The listing builds one solid part. Answer for the finished solid, in the listing's coordinates (mm). Face numbers are marked on the shaded views. A direction names the side the tool comes from. Round coordinates to 2 decimals unless told otherwise and drop trailing zeros. Write each loop counter-clockwise with the first axis right and the second up, starting at its lowest first coordinate (ties: lowest second). Pieces come first, ordered by that corner, then holes.
Item 1: Each of these flat-tipped pins is pushed along its axis until it touches: pin 1 (2 mm diameter, centred on x = 4, y = 13, fed in from -Z); pin 2 (1 mm diameter, centred on x = 2, y = 10, fed in from +Z); pin 3 (1.5 mm diameter, centred on x = -3, y = 2.5, fed in from +Z). Where does it stop, or does it pass through?
Item 2: Find section B-B on z = -5.5. Give the vertices of the cut face in (x, y), then the cut area to 3 significant figures.
Item 3: For a pull along Z with two mould halves and no side action, classify the marked faces 4 and 5 as +Z half, -Z half, draft (parallel to the pull), parting line (faces both ways), or undercut.
Item 4: Find section D-D on z = 0. Give the vertices of the cut face in (x, y).
Item 5: Find section C-C on x = 0. Give the vertices of the cut face in (y, z).
Item 6: Find section A-A on x = -4.25. Give the vertices of the cut face in (y, z), then the cut area to 3 significant figures.
Item 7: Find the intervals of material crossed by probe 1 along X at (y, z) = (10.5, -6.25); probe 2 along X at (y, z) = (7.75, -7); probe 3 along Z at (x, y) = (-6.5, 3), in increasing order.
Item 8: A tool of negligible diameter and unlimited length cuts with its end or side. For the marked faces 1, 2 and 3, from which of +Z, -Z, +X, -X, +Y, -Y can it reach the whole face along a straight path? Write none if from no direction.
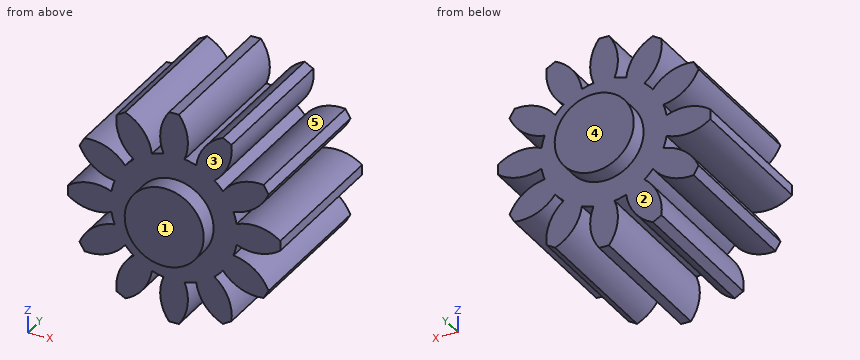
```python
from build123d import *

# Parameters (mm, degrees)
BOSS_EXTRUDE2_DEPTH = 12.5
CIRPATTERN1_COUNT   = 12


with BuildPart() as part:
    # Sketch1 → Revolve1 (revolve)
    with BuildSketch(Plane(origin=(0, 0, 0), x_dir=(0, 0, -1), z_dir=(1, 0, 0)), mode=Mode.PRIVATE) as revolve1_sk:
        Polygon((0, 0), (3.2, 0), (3.2, 1.5), (5.13, 1.5), (5.13, 14), (3.2, 14), (3.2, 15.5), (0, 15.5), align=None)
    revolve(revolve1_sk.sketch.rotate(Axis((0, 15.5, 0), (0, -1, 0)), 180), axis=Axis((0, 15.5, 0), (0, -1, 0)))

    # Sketch2 → Boss-Extrude2 (add)
    with BuildSketch(Plane(origin=(0, 14, 0), x_dir=(1, 0, 0), z_dir=(0, 1, 0))):
        with BuildLine():
            Line((0.4, 8.6), (-0.4, 8.6))
            ThreePointArc((-0.4, 8.6), (-1.094743674, 6.889243261), (-0.85, 5.059090827))
            Line((-0.85, 5.059090827), (-0.85, 4.768997596))
            Line((-0.85, 4.768997596), (0.85, 4.768997596))
            Line((0.85, 4.768997596), (0.85, 5.059090827))
            ThreePointArc((0.85, 5.059090827), (1.094743674, 6.889243261), (0.4, 8.6))
        make_face()
    boss_extrude2 = extrude(amount=-BOSS_EXTRUDE2_DEPTH)

    # CirPattern1: Boss-Extrude2 ×12 about axis
    cirpattern1_axis = Axis((0, 0, 0), (0, 1, 0))
    for i in range(1, CIRPATTERN1_COUNT):
        add(boss_extrude2.rotate(cirpattern1_axis, i * 360 / CIRPATTERN1_COUNT))


solid = part.part
```
Check values:
1. pin 1: stops at z = -7.65
1. pin 2: stops at z = 6.52
1. pin 3: stops at z = 7.55
2. outline: (-4.43, 1.5) - (-1.96, 1.5) - (-1.96, 14) - (-4.43, 14) - close; (-1, 1.5) - (1, 1.5) - (1, 14) - (-1, 14) - close; (1.96, 1.5) - (4.43, 1.5) - (4.43, 14) - (1.96, 14) - close
2. area: 86.7 mm2
3. face 4: draft
3. face 5: undercut
4. outline: (-8.6, 1.5) - (-3.2, 1.5) - (-3.2, 0) - (3.2, 0) - (3.2, 1.5) - (8.6, 1.5) - (8.6, 14) - (3.2, 14) - (3.2, 15.5) - (-3.2, 15.5) - (-3.2, 14) - (-8.6, 14) - close
5. outline: (0, -3.2) - (1.5, -3.2) - (1.5, -8.6) - (14, -8.6) - (14, -3.2) - (15.5, -3.2) - (15.5, 3.2) - (14, 3.2) - (14, 8.6) - (1.5, 8.6) - (1.5, 3.2) - (0, 3.2) - close
6. outline: (1.5, -7.48) - (14, -7.48) - (14, -5.12) - (1.5, -5.12) - close; (1.5, -3.6) - (14, -3.6) - (14, 3.6) - (1.5, 3.6) - close; (1.5, 5.12) - (14, 5.12) - (14, 7.48) - (1.5, 7.48) - close
6. area: 149 mm2
7. probe 1: x = -4.63 to -2.31, -1.12 to 1.12, 2.31 to 4.63
7. probe 2: x = -4.67 to -2.94, -1.08 to 1.08, 2.94 to 4.67
7. probe 3: z = -4.66 to -2.49, -1.12 to 1.12, 2.49 to 4.66
8. face 1: +Z, -Z, +X, -X, -Y
8. face 2: +Y
8. face 3: -Y
